Answer from the drawing. Dimensions are ordinates in mm from the lowest x, y and z of the part. Coordinates: 2 decimals unless noted, no trailing zeros.
(1) The part is cut by section A-A, the plane z = 6.5. State how many separate pieces and enclosed holes the cut face has, and give its area (3 significant figures).
(2) Straight lines are drawn through the part: line 1 along X through (y, z) = (11.25, 0.5) (1 decimal); line 2 along X through (y, z) = (12.75, 4.75) (1 decimal); line 3 along Y through (x, z) = (16, 1.25) (1 decimal). For each, find the intervals that lie inside material, in ascending order.
(3) Given pin 1 (1.5 mm diameter, centred on x = 10.04, y = 3.27, fed in from -Z); pin 2 (1 mm diameter, centred on y = 8.5, z = 2.5, fed in from +X); pin 3 (2 mm diameter, centred on y = 16.5, z = 5.5, fed in from -X) (1 decimal), each flat-ended and moving along its own axis, determine where each tip first touches the part or whether it passes through.
(4) Determine the mould class of the marked faces 1, 2 and 3 for opening direction Y: pulls with the +Y half, pulls with the -Y half, needs draft (parallel to the pull), parting line crosses it, or undercut.
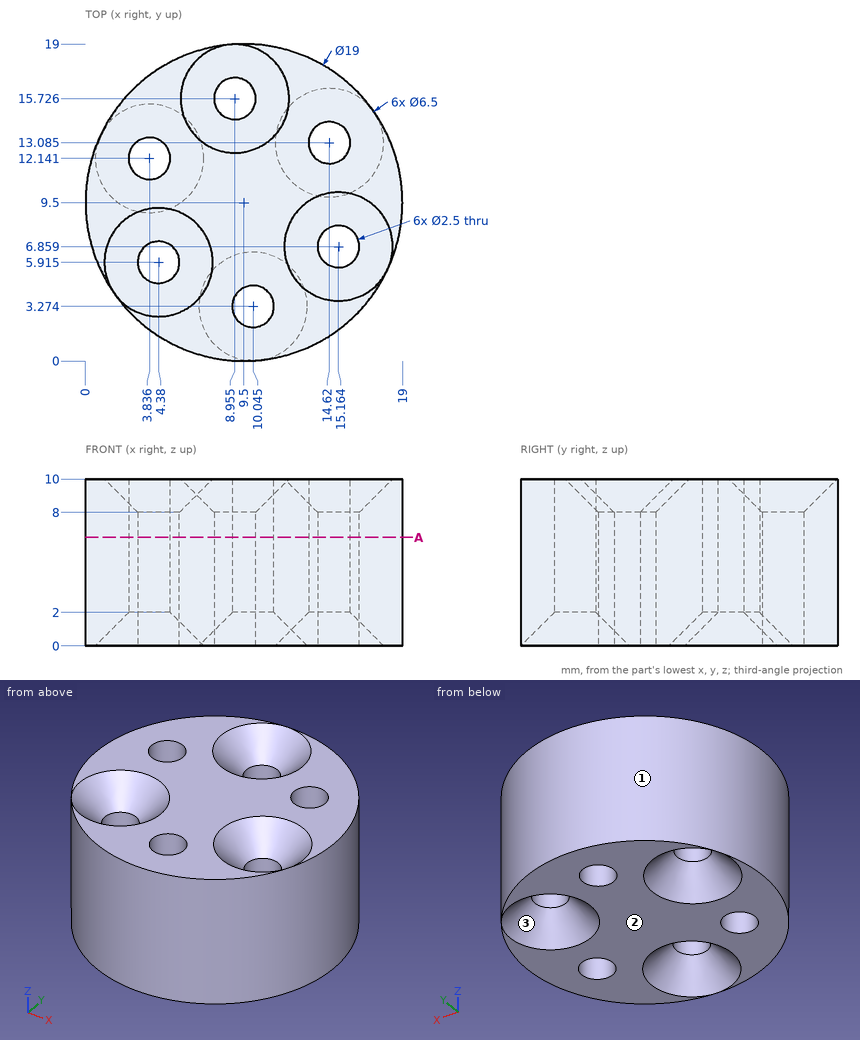
Computed:
1. separate pieces: 1
1. enclosed holes: 6
1. area: 254 mm2
2. line 1: x = 0.2 to 1.2, 6.4 to 12.6, 16.7 to 18.8
2. line 2: x = 0.6 to 2.7, 4.9 to 13.4, 15.8 to 18.4
2. line 3: y = 2.6 to 5.9, 7.8 to 11.6, 14.5 to 16.4
3. pin 1: passes through
3. pin 2: stops at x = 18.99
3. pin 3: stops at x = 2.1
4. face 1: parting line crosses it
4. face 2: needs draft
4. face 3: undercut
